Study the drawing (mm; zero at the part's minimum x, y, z) and answer. Coordinates: 2 decimals unless noted, no trailing zeros. Order: outer loops, then holes, each group sorted by start corner. A loop starts at its lowest first (then second) coordinate and runs counter-clockwise, first axis right, second up.
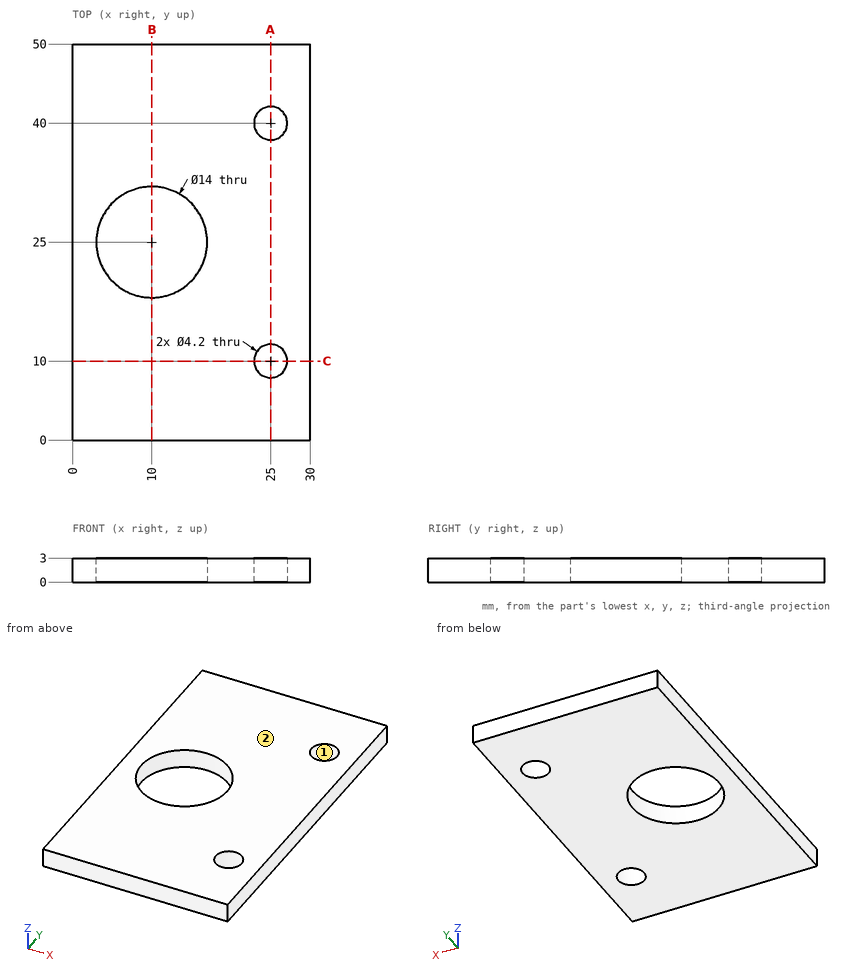
1) Straight lines are drawn through the part: line 1 (Y direction, x = 25, z = 1.5); line 2 (Y direction, x = 10, z = 2.35); line 3 (Y direction, x = 12.5, z = 1.6). For each, find the intervals that lie inside material, in ascending order.
A:
line 1: y = 0 to 7.9, 12.1 to 37.9, 42.1 to 50
line 2: y = 0 to 18, 32 to 50
line 3: y = 0 to 18.46, 31.54 to 50
2) A cutting plane is placed at A-A, the plane x = 25. Determine the outline of the cut face in (y, z).
A:
outline: (0, 0) - (7.9, 0) - (7.9, 3) - (0, 3) - close; (12.1, 0) - (37.9, 0) - (37.9, 3) - (12.1, 3) - close; (42.1, 0) - (50, 0) - (50, 3) - (42.1, 3) - close
3) A cutting plane is placed at B-B, the plane x = 10. Determine the outline of the cut face in (y, z).
A:
outline: (0, 0) - (18, 0) - (18, 3) - (0, 3) - close; (32, 0) - (50, 0) - (50, 3) - (32, 3) - close
4) A cutting plane is placed at C-C, the plane y = 10. Determine the outline of the cut face in (x, z).
A:
outline: (0, 0) - (22.9, 0) - (22.9, 3) - (0, 3) - close; (27.1, 0) - (30, 0) - (30, 3) - (27.1, 3) - close
5) A flat-ended cylindrical pin translates along its axis: pin 1 Ø6 at (x, y) = (12, 29) entering from -Z. Find the tip coordinate at first contact, or state that the pin passes through.
A:
pin 1: stops at z = 0
6) Determine the mould class of the marked faces 1 and 2 for opening direction Y: pulls with the +Y half, pulls with the -Y half, needs draft (parallel to the pull), parting line crosses it, or undercut.
A:
face 1: undercut
face 2: needs draft
